from build123d import *

# Parameters (mm, degrees)
SKETCH_2_R      = 0.85
SKETCH_2_R_2    = 1.75
EXTRUDE_1_DEPTH = 1.5


with BuildPart() as part:
    # 草图2 → 凸台-拉伸1 (new body)
    with BuildSketch(Plane(origin=(0, 7.096792112, 0), x_dir=(1, 0, 0), z_dir=(0, 1, 0))):
        Polygon((-1.9, 0), (-10.4, 0), (-10.4, -1.5), (-9.4, -1.5), (-9.4, -1), (-9.1, -1), (-8.4, -1.5), (1.371788561, -1.5), (5.355505418, 0.8), (13.1, 0.8), (13.1, 5.8), (-1.303412873, 5.8), (-2.936751866, 3.3), (-8.4, 3.3), (-8.4, 0.8), (-1.9, 0.8), align=None)
        with Locations(Location((11.1, 3.3, 0), (0, 0, 180))):
            Circle(SKETCH_2_R, mode=Mode.SUBTRACT)
        with Locations(Location((0.6, 3.3, 0), (0, 0, 180))):
            Circle(SKETCH_2_R_2, mode=Mode.SUBTRACT)
    extrude(amount=-EXTRUDE_1_DEPTH)


solid = part.part
Read the model definition and answer for the solid it produces. Units are mm, in the model's axes. A direction names the side the tool comes from. Give positions to 0.01 mm unless a question says otherwise; leave off trailing zeros. Write each loop counter-clockwise with the first axis right and the second up, starting at its lowest first coordinate (ties: lowest second). Pieces come first, ordered by that corner, then holes. Notation, with made-up numbers: (11, 24.5) -> (44, 24.5) arc R30 ccw to (44, 47.5) -> close; hole circle Ø2 at (-29.75, 1.25). An arc over 180 degrees is marked (long way). Answer as a JSON object with one key per item and string values. Group by question number.
1) Find section C-C (z = -2). Write down the section's boundary in (x, y).
2) Each of these flat-tipped pins is pushed along its axis until it touches: P1, Ø1, axis at x = 7, z = 0.5, coming from the -Y side; P2, Ø0.8, axis at y = 6.5, z = -2, coming from the -X side; P3, Ø3, axis at x = 1, z = -4.5, coming from the -Y side. Where does it stop, or does it pass through?
3) Find section D-D (x = 6.5). Write down the section's boundary in (y, z).
4) The mould has two halves that part along X. Classify faces 1 (the flat face through (3.336, 6.357, 0.366)), 2 (the cylindrical face through (0.98, 6.36, -5.01)), 3 (the flat face through (-6, 6, -3.3)): +X half, -X half, draft (parallel to the pull), parting line (faces both ways), or undercut.
5) A tool of negligible diameter and unlimited length cuts with its end or side. For faces 4 (the flat face through (-8.4, 6, -2)), 5 (the flat face through (1, 5.597, -1)), 6 (the flat face through (-6, 6, 0)), 7 (the flat face through (9, 6, -0.8)), from which of +Z, -Z, +X, -X, +Y, -Y can it reach the whole face along a straight path? Write none if from no direction.
6) Find section B-B (y = 6.2). Write down the section's boundary in (x, z), and give its area (3 significant figures).
7) Find section A-A (x = 0.6). Write down the section's boundary in (y, z).
8) Consider L1, parallel to Z at x = 11.1, y = 6.5; L2, parallel to Z at x = 0.6, y = 6.1; L3, parallel to X at y = 6.3, z = -2.75. Determine where each line is inside the solid, lowest interval first. Write a range as from..to.
Values follow:
{
 "1": {"outline": "(-8.4, 5.6) -> (-0.57, 5.6) -> (-0.57, 7.1) -> (-8.4, 7.1) -> close; (1.77, 5.6) -> (13.1, 5.6) -> (13.1, 7.1) -> (1.77, 7.1) -> close"},
 "2": {"P1": "passes through", "P2": "stops at x = -8.4", "P3": "stops at y = 5.6"},
 "3": {"outline": "(5.6, -5.8) -> (7.1, -5.8) -> (7.1, -0.8) -> (5.6, -0.8) -> close"},
 "4": {"face 1": "+X half", "face 2": "undercut", "face 3": "draft"},
 "5": {"face 4": "-Z, -X, +Y, -Y", "face 5": "+Z, -Z, +X, -X, -Y", "face 6": "-X, +Y, -Y", "face 7": "+Z, +X, +Y, -Y"},
 "6": {"outline": "(-10.4, 0) -> (-1.9, 0) -> (-1.9, -0.8) -> (-8.4, -0.8) -> (-8.4, -3.3) -> (-2.94, -3.3) -> (-1.3, -5.8) -> (13.1, -5.8) -> (13.1, -0.8) -> (5.36, -0.8) -> (1.37, 1.5) -> (-8.4, 1.5) -> (-9.1, 1) -> (-9.4, 1) -> (-9.4, 1.5) -> (-10.4, 1.5) -> close; hole circle Ø3.5 at (0.6, -3.3); hole circle Ø1.7 at (11.1, -3.3)", "area": "104 mm2"},
 "7": {"outline": "(5.6, -5.8) -> (7.1, -5.8) -> (7.1, -5.05) -> (5.6, -5.05) -> close; (5.6, -1.55) -> (7.1, -1.55) -> (7.1, 1.5) -> (5.6, 1.5) -> close"},
 "8": {"L1": "z = -5.8..-4.15, -2.45..-0.8", "L2": "z = -5.8..-5.05, -1.55..1.5", "L3": "x = -8.4..-1.06, 2.26..10.45, 11.75..13.1"}
}
